For this review, take the finished solid that the model builds, in its own axes (mm). A direction names the side the tool comes from. Give positions to 0.01 mm unless a question says otherwise; leave off trailing zeros. Write each loop counter-clockwise with the first axis right and the second up, starting at its lowest first coordinate (ties: lowest second). Pieces come first, ordered by that corner, then holes. Notation, with made-up numbers: (-35, 32) -> (19, 32) arc R12 ccw to (19, 54) -> close; hole circle Ø10 at (46.5, 23.25). An arc over 180 degrees is marked (long way). Return JSON: item names as keys, results as strings.
from build123d import *

# Parameters (mm, degrees)
BOSS_EXTRUDE1_DEPTH = 3
SKETCH3_R           = 2.1
CUT_EXTRUDE1_DEPTH  = 3
FILLET1_R           = 3


with BuildPart() as part:
    # Sketch1 → Revolve1 (revolve)
    with BuildSketch(Plane.XY, mode=Mode.PRIVATE) as revolve1_sk:
        Polygon((73.5, 0), (75, 0), (106.5, 80), (103.5, 80), align=None)
    revolve(revolve1_sk.sketch.rotate(Axis((0, 0, 0), (0, 1, 0)), 90), axis=Axis((0, 0, 0), (0, 1, 0)))

    # Sketch2 → Boss-Extrude1 (add)
    with BuildSketch(Plane.XZ):
        with BuildLine():
            Line((72.284161474, -20), (95, -20))
            Line((95, -20), (95, 20))
            Line((95, 20), (72.284161474, 20))
            ThreePointArc((72.284161474, 20), (75, 0), (72.284161474, -20))
        make_face()
        with BuildLine():
            Line((-95, 20), (-72.284161474, 20))
            ThreePointArc((-72.284161474, 20), (-75, 0), (-72.284161474, -20))
            Line((-72.284161474, -20), (-95, -20))
            Line((-95, -20), (-95, 20))
        make_face()
    extrude(amount=-BOSS_EXTRUDE1_DEPTH)

    # Sketch3 → Cut-Extrude1 (cut)
    with BuildSketch(Plane.XZ):
        with Locations(Location((85, 10, 0), (0, 0, 270))):
            Circle(SKETCH3_R)
        with Locations(Location((85, -10, 0), (0, 0, 90))):
            Circle(SKETCH3_R)
        with Locations(Location((-85, -10, 0), (0, 0, 270))):
            Circle(SKETCH3_R)
        with Locations(Location((-85, 10, 0), (0, 0, 90))):
            Circle(SKETCH3_R)
    extrude(amount=-CUT_EXTRUDE1_DEPTH, mode=Mode.SUBTRACT)

    # Fillet1
    fillet1_edges = [part.edges().sort_by_distance(p)[0] for p in [
        (76.18125, 3, 0),
        (-76.18125, 3, 0),
    ]]
    fillet(fillet1_edges, radius=FILLET1_R)


solid = part.part
1. Add section A-A, the plane z = 0. State the section outline as (x, y) points, plus the area to 3 significant figures.
Results found:
{"outline": "(-106.5, 80) -> (-77.8, 7.1) arc R3 cw to (-80.59, 3) -> (-95, 3) -> (-95, 0) -> (-73.5, 0) -> (-103.5, 80) -> close; (73.5, 0) -> (95, 0) -> (95, 3) -> (80.59, 3) arc R3 cw to (77.8, 7.1) -> (106.5, 80) -> (103.5, 80) -> close", "area": "485 mm²"}
2. The part is to be moulded in two halves that separate along X. For faces 5 (the conical face through (30.821, 13.893, -74.334)), 6 (the flat face through (84, 2, 20)), 7 (the conical face through (47.638, 12.773, 62.128)), say which applies: +X half, -X half, draft (parallel to the pull), parting line (faces both ways), or undercut.
Results found:
{"face 5": "parting line", "face 6": "draft", "face 7": "undercut"}
3. For pin 1 (2 mm diameter, centred on x = 74.5, y = 29, fed in from -Z); pin 2 (10 mm diameter, centred on y = 43, z = -56, fed in from -X); pin 3 (1 mm diameter, centred on y = 54.5, z = -33.5, fed in from -X), all flat-tipped, find the tip position at first contact; note any pin that passes through.
Results found:
{"pin 1": "stops at z = -45.62", "pin 2": "stops at x = -77.24", "pin 3": "stops at x = -90.73"}
4. For faces 1 (the flat face through (-84, 2, 20)), 2 (the flat face through (-83, 2, -20)), 3 (the flat face through (-103, 80, 16)), 4 (the flat face through (83, 2, -20)), list the 3-axis set-ups (+Z, -Z, +X, -X, +Y, -Y) from which the entire face can be reached by the end or side of a thin tool; tool diameter is ignored.
Results found:
{"face 1": "+Z, -X, -Y", "face 2": "-Z, -X, -Y", "face 3": "+Z, -Z, +X, -X, +Y", "face 4": "-Z, +X, -Y"}
5. Add section C-C, the plane y = 55.5. State the section outline as (x, z) points (1 decimal).
Results found:
{"outline": "circle Ø193.7 at (0, 0); hole circle Ø188.6 at (0, 0)"}
6. To check wall thickness, follow probe 1 along X at (y, z) = (2, -10); probe 2 along X at (y, z) = (1.35, -10); probe 3 along Z at (x, y) = (60, 67.5). State the ranges of each line that lie inside material, in increasing order.
Results found:
{"probe 1": "x = -95 to -87.1, -82.9 to -73.57, 73.57 to 82.9, 87.1 to 95", "probe 2": "x = -95 to -87.1, -82.9 to -73.33, 73.33 to 82.9, 87.1 to 95", "probe 3": "z = -81.96 to -78.51, 78.51 to 81.96"}
7. Add section B-B, the plane y = 69.5. State the section outline as (x, z) points (1 decimal).
Results found:
{"outline": "circle Ø204.7 at (0, 0); hole circle Ø199.1 at (0, 0)"}
